Work out the finished part from the listing and answer in its coordinate system (mm). A direction names the side the tool comes from. Coordinates: 2 decimals unless noted, no trailing zeros. Loops run counter-clockwise (first coordinate to the right, second up) from the corner with the lowest first, then second, coordinate; pieces in that order, holes last. Notation, with made-up numbers: (28.25, 5) -> (51.25, 5) arc R12 cw to (51.25, 9) -> close; hole circle Ø11 at (56.25, 71). An arc over 180 degrees is marked (long way). Use a Markdown table: item, result.
from build123d import *

# Parameters (mm, degrees)
SKETCH1_R           = 3
BOSS_EXTRUDE1_DEPTH = 11.938
SKETCH2_R           = 0.9779
BOSS_EXTRUDE2_DEPTH = 5.2832
BOSS_EXTRUDE3_DEPTH = 4.2418


with BuildPart() as part:
    # Sketch1 → Boss-Extrude1 (new body)
    with BuildSketch(Plane(origin=(0, 0, 0), x_dir=(1, 0, 0), z_dir=(0, 1, 0))):
        Circle(SKETCH1_R)
    extrude(amount=BOSS_EXTRUDE1_DEPTH)

    # Sketch2 → Boss-Extrude2 (add)
    with BuildSketch(Plane(origin=(0, 11.938, 0), x_dir=(1, 0, 0), z_dir=(0, 1, 0))):
        Circle(SKETCH2_R)
    extrude(amount=BOSS_EXTRUDE2_DEPTH)

    # Sketch4 → Boss-Extrude3 (add)
    with BuildSketch(Plane(origin=(0, 17.2212, -17.2212), x_dir=(1, 0, 0), z_dir=(0, -1, 0))):
        with BuildLine():
            Line((0, 20.1041), (0, 18.4912))
            ThreePointArc((0, 18.4912), (1.27, 17.2212), (0, 15.9512))
            Line((0, 15.9512), (0, 14.3383))
            ThreePointArc((0, 14.3383), (-2.8829, 17.2212), (0, 20.1041))
        make_face()
    extrude(amount=BOSS_EXTRUDE3_DEPTH)


solid = part.part
Q1. Section A-A on x = -1.8 is taken. Determine the outline of the cut face in (y, z).
Solved:
| item | result |
|---|---|
| outline | (0, -2.4) -> (11.94, -2.4) -> (11.94, 2.4) -> (0, 2.4) -> close; (12.98, -2.25) -> (17.22, -2.25) -> (17.22, 2.25) -> (12.98, 2.25) -> close |
Q2. Section D-D on x = -0.8 is taken. Determine the outline of the cut face in (y, z).
Solved:
| item | result |
|---|---|
| outline | (0, -2.89) -> (11.94, -2.89) -> (11.94, -0.56) -> (12.98, -0.56) -> (12.98, -2.77) -> (17.22, -2.77) -> (17.22, 2.77) -> (12.98, 2.77) -> (12.98, 0.56) -> (11.94, 0.56) -> (11.94, 2.89) -> (0, 2.89) -> close |
Q3. For faces 4 (the cylindrical face through (1.27, 15.13, 0.03)), 5 (the flat face through (-1, 11.938, -1)), 6 (the flat face through (0, 15, 2)), determine the directions among +Z, -Z, +X, -X, +Y, -Y from which every point of the face is accessible in a straight line to the end or side of a thin tool.
Solved:
| item | result |
|---|---|
| face 4 | +X, +Y |
| face 5 | none |
| face 6 | +Z, +X, +Y |
Q4. Section C-C on y = 3.75 is taken. Determine the outline of the cut face in (x, z), and give its area (3 significant figures).
Solved:
| item | result |
|---|---|
| outline | circle Ø6 at (0, 0) |
| area | 28.3 mm² |
Q5. Determine the mould class of faces 1 (the cylindrical face through (0.933, 12.451, -0.294)), 2 (the flat face through (0, 15, -2)), 3 (the flat face through (-1, 17.221, 0)) for opening direction Y: pulls with the +Y half, pulls with the -Y half, needs draft (parallel to the pull), parting line crosses it, or undercut.
Solved:
| item | result |
|---|---|
| face 1 | undercut |
| face 2 | needs draft |
| face 3 | pulls with the +Y half |
Q6. Consider line 1 (Y direction, x = 1.2, z = -0.05); line 2 (Z direction, x = -0.05, y = 12.5); line 3 (Y direction, x = 1.4, z = 1.15). Determine where each line is inside the solid, lowest interval first. Write a range as [from, to].
Solved:
| item | result |
|---|---|
| line 1 | [0, 11.94], [12.98, 17.22] |
| line 2 | [-0.98, 0.98] |
| line 3 | [0, 11.94] |
Q7. Given pin 1 Ø0.5 at (y, z) = (14, -2.5) entering from +X; pin 2 Ø2 at (x, y) = (-2, 15.5) entering from -Z; pin 3 Ø1.2 at (x, z) = (-0.5, -1) entering from -Y; pin 4 Ø2 at (x, y) = (1.5, 5) entering from +Z, each flat-ended and moving along its own axis, determine where each tip first touches the part or whether it passes through.
Solved:
| item | result |
|---|---|
| pin 1 | x = 0 |
| pin 2 | z = -2.7 |
| pin 3 | y = 0 |
| pin 4 | z = 2.96 |
Q8. Section B-B on z = 0 is taken. Determine the outline of the cut face in (x, y), and give its area (3 significant figures).
Solved:
| item | result |
|---|---|
| outline | (-3, 0) -> (3, 0) -> (3, 11.94) -> (0.98, 11.94) -> (0.98, 12.98) -> (1.27, 12.98) -> (1.27, 17.22) -> (-2.88, 17.22) -> (-2.88, 12.98) -> (-0.98, 12.98) -> (-0.98, 11.94) -> (-3, 11.94) -> close |
| area | 91.3 mm² |
